from build123d import *

# Parameters (mm, degrees)
BOSS_EXTRUDE1_DEPTH    = 10
BOSS_EXTRUDE2_DEPTH    = 15
F_25_0MM_DOWEL_HOLE1_D = 25


with BuildPart() as part:
    # Sketch2 → Boss-Extrude1 (new body)
    with BuildSketch(Plane(origin=(0, 0, 0), x_dir=(1, 0, 0), z_dir=(0, 1, 0))):
        Polygon((0, 0), (100.00000548, 0), (100, -200), (0, -200.00001096), align=None)
    extrude(amount=BOSS_EXTRUDE1_DEPTH)

    # Sketch3 → Boss-Extrude2 (add)
    with BuildSketch(Plane(origin=(0.867898509, 10, -1.693868364), x_dir=(1, 0, 0), z_dir=(0, 1, 0))):
        Polygon((59.097520158, -1.533073759), (59.097520158, -61.533073759), (99.097520158, -61.533073759), (99.866800969, -1.533073759), align=None)
    extrude(amount=BOSS_EXTRUDE2_DEPTH)

    # Ø25.0mm Dowel Hole1 (through all)
    with Locations(Plane(origin=(0, 10, 0), x_dir=(1, 0, 0), z_dir=(0, 1, 0))):
        with Locations((65, -170)):
            Hole(F_25_0MM_DOWEL_HOLE1_D / 2)


solid = part.part
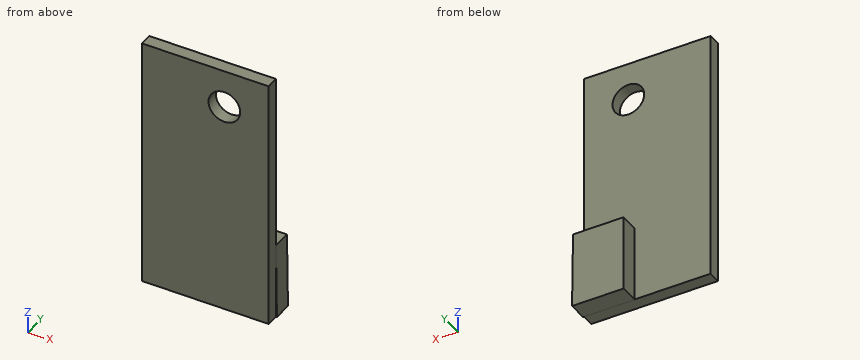
The model under review builds one solid part; all positions refer to its coordinate system, in mm. Round coordinates to 2 decimals unless told otherwise and drop trailing zeros. Order: outer loops, then holes, each group sorted by start corner. A loop starts at its lowest first (then second) coordinate and runs counter-clockwise, first axis right, second up. Notation, with made-up numbers: (47, 62.5) -> (84, 62.5) arc R26 cw to (84, 92.5) -> close; hole circle Ø8 at (-37.75, -23). An arc over 180 degrees is marked (long way). Return JSON: item names as keys, results as strings.
1. Take a section at B-B (z = 170). Write out the cut boundary in (x, y).
Answer block:
{"outline": "(0, 0) -> (52.5, 0) -> (52.5, 10) -> (0, 10) -> close; (77.5, 0) -> (100, 0) -> (100, 10) -> (77.5, 10) -> close"}
2. Take a section at D-D (z = 21). Write out the cut boundary in (x, y), then the cut area to 3 significant figures.
Answer block:
{"outline": "(0, 0) -> (100, 0) -> (100, 10) -> (100.46, 10) -> (100.46, 25) -> (59.97, 25) -> (59.97, 10) -> (0, 10) -> close", "area": "1,610 mm²"}
3. Take a section at A-A (x = 75). Write out the cut boundary in (y, z).
Answer block:
{"outline": "(0, 0) -> (10, 0) -> (10, -0.16) -> (25, -0.16) -> (25, 59.84) -> (10, 59.84) -> (10, 162.5) -> (0, 162.5) -> close; (0, 177.5) -> (10, 177.5) -> (10, 200) -> (0, 200) -> close"}
4. Insertion check: P1, Ø4, axis at x = 27, y = 10, coming from the -Z side; P2, Ø1.5, axis at y = 11, z = 47, coming from the -X side; P3, Ø1, axis at x = 54.5, z = 58, coming from the +Y side; P4, Ø15, axis at x = 65, z = 170, coming from the -Y side. Each pin has a flat end and moves straight along its axis. Give the tip position at first contact, or say it passes through.
Answer block:
{"P1": "stops at z = 0", "P2": "stops at x = 59.97", "P3": "stops at y = 10", "P4": "passes through"}
5. For L1, parallel to Z at x = 65, y = 2.5; L2, parallel to X at y = 2.5, z = 170; L3, parallel to Y at x = 63.5, z = 150.5, list the stretches that pass through material, from the lowest coordinate up. Write a range as [from, to].
Answer block:
{"L1": "z = [0, 157.5], [182.5, 200]", "L2": "x = [0, 52.5], [77.5, 100]", "L3": "y = [0, 10]"}
6. Take a section at C-C (y = 2.5). Write out the cut boundary in (x, z), then the cut area to 3 significant figures.
Answer block:
{"outline": "(0, 0) -> (100, 0) -> (100, 200) -> (0, 200) -> close; hole circle Ø25 at (65, 170)", "area": "19,500 mm²"}
